```python
from build123d import *

# Parameters (mm, degrees)
SKETCH1_W                 = 50.11
SKETCH1_H                 = 43.44
BOSS_EXTRUDE1_DEPTH       = 97.79
SKETCH2_W                 = 23.32
SKETCH2_H                 = 45.06
CUT_EXTRUDE1_DEPTH        = 119.156378584
SHELL1_T                  = -2
SHELL1_THICKNESS_2_FACE_W = 39.44
SHELL1_THICKNESS_2_FACE_H = 22.79
SHELL1_THICKNESS_2_DEPTH  = 18.02
SKETCH4_W                 = 6.5
SKETCH4_H                 = 11
CUT_EXTRUDE2_DEPTH        = 2
SKETCH6_R                 = 2
CUT_EXTRUDE3_DEPTH        = 2
CUT_EXTRUDE5_DEPTH        = 2
SKETCH8_R                 = 8.25
CUT_EXTRUDE6_DEPTH        = 20.02
FILLET1_R                 = 10
FILLET2_R                 = 2


with BuildPart() as part:
    # Sketch1 → Boss-Extrude1 (new body)
    with BuildSketch(Plane(origin=(0, 0, 0), x_dir=(1, 0, 0), z_dir=(0, 1, 0))):
        with Locations((25.055, 21.72)):
            Rectangle(SKETCH1_W, SKETCH1_H)
    extrude(amount=BOSS_EXTRUDE1_DEPTH)

    # Sketch2 → Cut-Extrude1 (cut, through all)
    with BuildSketch(Plane.XY):
        with Locations((11.66, 22.53)):
            Rectangle(SKETCH2_W, SKETCH2_H)
    extrude(amount=-CUT_EXTRUDE1_DEPTH, mode=Mode.SUBTRACT)

    # Shell1
    shell1_openings = [part.faces().sort_by_distance(p)[0] for p in [
        (25.055, 97.79, -21.72),
    ]]
    offset(amount=SHELL1_T, openings=shell1_openings, kind=Kind.INTERSECTION)

    # Shell1 thickness 2 face (on inner face of the shell) → Shell1 thickness 2 (add)
    with BuildSketch(Plane(origin=(36.715, 2, -21.72), x_dir=(0, 0, -1), z_dir=(0, -1, 0))):
        Rectangle(SHELL1_THICKNESS_2_FACE_W, SHELL1_THICKNESS_2_FACE_H)
    extrude(amount=-SHELL1_THICKNESS_2_DEPTH)

    # Sketch4 → Cut-Extrude2 (cut)
    with BuildSketch(Plane.XZ.offset(-45.06)):
        with Locations((4.35, -30.69)):
            Rectangle(SKETCH4_W, SKETCH4_H)
    extrude(amount=-CUT_EXTRUDE2_DEPTH, mode=Mode.SUBTRACT)

    # Sketch6 → Cut-Extrude3 (cut)
    with BuildSketch(Plane.XY):
        with Locations((44.415, 88.885)):
            Circle(SKETCH6_R)
        with Locations((25.815, 88.885)):
            Circle(SKETCH6_R)
        with Locations((44.415, 53.805)):
            Circle(SKETCH6_R)
        with Locations((25.815, 53.805)):
            Circle(SKETCH6_R)
    extrude(amount=-CUT_EXTRUDE3_DEPTH, mode=Mode.SUBTRACT)

    # Sketch7 → Cut-Extrude5 (cut)
    with BuildSketch(Plane(origin=(0, 0, 0), x_dir=(0, 0, -1), z_dir=(1, 0, 0))):
        with BuildLine():
            Line((22.64, 91.29), (22.64, 97.79))
            Line((22.64, 97.79), (11.64, 97.79))
            Line((11.64, 97.79), (11.64, 91.29))
            ThreePointArc((11.64, 91.29), (17.14, 85.79), (22.64, 91.29))
        make_face()
    extrude(amount=CUT_EXTRUDE5_DEPTH, mode=Mode.SUBTRACT)

    # Sketch8 → Cut-Extrude6 (cut)
    with BuildSketch(Plane(origin=(0, 0, 0), x_dir=(1, 0, 0), z_dir=(0, 1, 0))):
        with Locations(Location((36.715, 21.72, 0), (0, 0, 90))):
            Circle(SKETCH8_R)
    extrude(amount=CUT_EXTRUDE6_DEPTH, mode=Mode.SUBTRACT)

    # Fillet1
    fillet1_edges = [part.edges().sort_by_distance(p)[0] for p in [
        (23.32, 45.06, -21.72),
    ]]
    fillet(fillet1_edges, radius=FILLET1_R)

    # Fillet2
    # the kernel refuses this fillet: 2 mm, written as the material it takes off along each edge
    with BuildSketch(Plane(origin=(2, 47.06, -2), x_dir=(0, -1, 0), z_dir=(0, 0, 1))) as fillet2_piece_1_section:
        Polygon((0, 0), (FILLET2_R, 0), (FILLET2_R, -FILLET2_R), (0, -FILLET2_R), align=None)
    fillet2_piece_1 = extrude(amount=FILLET2_R, mode=Mode.PRIVATE)
    fillet2_piece_1 = fillet2_piece_1 - Plane(origin=(2, 47.06, -2), x_dir=(0.7071067811865475, 0.7071067811865475, 0), z_dir=(0, 0, 1)) * Sphere(FILLET2_R, mode=Mode.PRIVATE)
    add(fillet2_piece_1, mode=Mode.SUBTRACT)
    with BuildSketch(Plane(origin=(2, 47.06, -41.44), x_dir=(-1, 0, 0), z_dir=(0, -1, 0))) as fillet2_piece_2_section:
        Polygon((0, 0), (FILLET2_R, 0), (FILLET2_R, FILLET2_R), (0, FILLET2_R), align=None)
    fillet2_piece_2 = extrude(amount=FILLET2_R, mode=Mode.PRIVATE)
    fillet2_piece_2 = fillet2_piece_2 - Plane(origin=(2, 47.06, -41.44), x_dir=(0.7071067811865475, 0, 0.7071067811865475), z_dir=(0, -1, 0)) * Sphere(FILLET2_R, mode=Mode.PRIVATE)
    add(fillet2_piece_2, mode=Mode.SUBTRACT)
    with BuildSketch(Plane(origin=(2, 95.79, -2), x_dir=(-1, 0, 0), z_dir=(0, 0, 1))) as fillet2_piece_3_section:
        Polygon((0, 0), (FILLET2_R, 0), (FILLET2_R, -FILLET2_R), (0, -FILLET2_R), align=None)
    fillet2_piece_3 = extrude(amount=FILLET2_R, mode=Mode.PRIVATE)
    fillet2_piece_3 = fillet2_piece_3 - Plane(origin=(2, 95.79, -2), x_dir=(0.7071067811865475, -0.7071067811865475, 0), z_dir=(0, 0, 1)) * Sphere(FILLET2_R, mode=Mode.PRIVATE)
    add(fillet2_piece_3, mode=Mode.SUBTRACT)
    with BuildSketch(Plane(origin=(2, 95.79, -41.44), x_dir=(0, 0, -1), z_dir=(-1, 0, 0))) as fillet2_piece_4_section:
        Polygon((0, 0), (FILLET2_R, 0), (FILLET2_R, -FILLET2_R), (0, -FILLET2_R), align=None)
    fillet2_piece_4 = extrude(amount=FILLET2_R, mode=Mode.PRIVATE)
    fillet2_piece_4 = fillet2_piece_4 - Plane(origin=(2, 95.79, -41.44), x_dir=(0, -0.7071067811865475, 0.7071067811865475), z_dir=(-1, 0, 0)) * Sphere(FILLET2_R, mode=Mode.PRIVATE)
    add(fillet2_piece_4, mode=Mode.SUBTRACT)
    with BuildSketch(Plane(origin=(25.32, 2, -2), x_dir=(-1, 0, 0), z_dir=(0, 0, 1))) as fillet2_piece_5_section:
        Polygon((0, 0), (FILLET2_R, 0), (FILLET2_R, FILLET2_R), (0, FILLET2_R), align=None)
    fillet2_piece_5 = extrude(amount=FILLET2_R, mode=Mode.PRIVATE)
    fillet2_piece_5 = fillet2_piece_5 - Plane(origin=(25.32, 2, -2), x_dir=(0.7071067811865475, 0.7071067811865475, 0), z_dir=(0, 0, 1)) * Sphere(FILLET2_R, mode=Mode.PRIVATE)
    add(fillet2_piece_5, mode=Mode.SUBTRACT)
    with BuildSketch(Plane(origin=(25.32, 2, -41.44), x_dir=(0, 0, -1), z_dir=(-1, 0, 0))) as fillet2_piece_6_section:
        Polygon((0, 0), (FILLET2_R, 0), (FILLET2_R, FILLET2_R), (0, FILLET2_R), align=None)
    fillet2_piece_6 = extrude(amount=FILLET2_R, mode=Mode.PRIVATE)
    fillet2_piece_6 = fillet2_piece_6 - Plane(origin=(25.32, 2, -41.44), x_dir=(0, 0.7071067811865475, 0.7071067811865475), z_dir=(-1, 0, 0)) * Sphere(FILLET2_R, mode=Mode.PRIVATE)
    add(fillet2_piece_6, mode=Mode.SUBTRACT)
    with BuildSketch(Plane(origin=(48.11, 2, -2), x_dir=(0, -1, 0), z_dir=(0, 0, 1))) as fillet2_piece_7_section:
        Polygon((0, 0), (FILLET2_R, 0), (FILLET2_R, FILLET2_R), (0, FILLET2_R), align=None)
    fillet2_piece_7 = extrude(amount=FILLET2_R, mode=Mode.PRIVATE)
    fillet2_piece_7 = fillet2_piece_7 - Plane(origin=(48.11, 2, -2), x_dir=(-0.7071067811865475, 0.7071067811865475, 0), z_dir=(0, 0, 1)) * Sphere(FILLET2_R, mode=Mode.PRIVATE)
    add(fillet2_piece_7, mode=Mode.SUBTRACT)
    with BuildSketch(Plane(origin=(48.11, 95.79, -2), x_dir=(0, 1, 0), z_dir=(0, 0, 1))) as fillet2_piece_8_section:
        Polygon((0, 0), (FILLET2_R, 0), (FILLET2_R, -FILLET2_R), (0, -FILLET2_R), align=None)
    fillet2_piece_8 = extrude(amount=FILLET2_R, mode=Mode.PRIVATE)
    fillet2_piece_8 = fillet2_piece_8 - Plane(origin=(48.11, 95.79, -2), x_dir=(-0.7071067811865475, -0.7071067811865475, 0), z_dir=(0, 0, 1)) * Sphere(FILLET2_R, mode=Mode.PRIVATE)
    add(fillet2_piece_8, mode=Mode.SUBTRACT)
    with BuildSketch(Plane(origin=(48.11, 95.79, -41.44), x_dir=(0, 1, 0), z_dir=(0, 0, -1))) as fillet2_piece_9_section:
        Polygon((0, 0), (FILLET2_R, 0), (FILLET2_R, FILLET2_R), (0, FILLET2_R), align=None)
    fillet2_piece_9 = extrude(amount=FILLET2_R, mode=Mode.PRIVATE)
    fillet2_piece_9 = fillet2_piece_9 - Plane(origin=(48.11, 95.79, -41.44), x_dir=(-0.7071067811865475, -0.7071067811865475, 0), z_dir=(0, 0, -1)) * Sphere(FILLET2_R, mode=Mode.PRIVATE)
    add(fillet2_piece_9, mode=Mode.SUBTRACT)
    with BuildSketch(Plane(origin=(48.11, 2, -41.44), x_dir=(0, -1, 0), z_dir=(0, 0, -1))) as fillet2_piece_10_section:
        Polygon((0, 0), (FILLET2_R, 0), (FILLET2_R, -FILLET2_R), (0, -FILLET2_R), align=None)
    fillet2_piece_10 = extrude(amount=FILLET2_R, mode=Mode.PRIVATE)
    fillet2_piece_10 = fillet2_piece_10 - Plane(origin=(48.11, 2, -41.44), x_dir=(-0.7071067811865475, 0.7071067811865475, 0), z_dir=(0, 0, -1)) * Sphere(FILLET2_R, mode=Mode.PRIVATE)
    add(fillet2_piece_10, mode=Mode.SUBTRACT)
    with BuildSketch(Plane(origin=(0, 45.06, -2), x_dir=(1, 0, 0), z_dir=(0, 0, -1)), Plane(origin=(50.11, 97.79, -2), x_dir=(-1, 0, 0), z_dir=(0, 0, -1))) as fillet2_piece_11:
        with BuildLine():
            CenterArc((FILLET2_R, -FILLET2_R), FILLET2_R, 90, 90)
            Line((0, -FILLET2_R), (0, 0))
            Line((0, 0), (FILLET2_R, 0))
        make_face()
    extrude(amount=39.44, mode=Mode.SUBTRACT)
    with BuildSketch(Plane(origin=(0, 97.79, -16.64), x_dir=(0, -1, 0), z_dir=(0, 0, 1))) as fillet2_piece_12:
        with BuildLine():
            CenterArc((FILLET2_R, FILLET2_R), FILLET2_R, 180, 90)
            Line((0, FILLET2_R), (0, 0))
            Line((0, 0), (FILLET2_R, 0))
        make_face()
    extrude(amount=14.64, mode=Mode.SUBTRACT)
    with BuildSketch(Plane(origin=(0, 47.06, 0), x_dir=(1, 0, 0), z_dir=(0, 1, 0)), Plane(origin=(0, 47.06, -43.44), x_dir=(0, 0, 1), z_dir=(0, 1, 0))) as fillet2_piece_13:
        with BuildLine():
            CenterArc((FILLET2_R, FILLET2_R), FILLET2_R, 180, 90)
            Line((0, FILLET2_R), (0, 0))
            Line((0, 0), (FILLET2_R, 0))
        make_face()
    extrude(amount=48.73, mode=Mode.SUBTRACT)
    with BuildSketch(Plane(origin=(0, 97.79, -41.44), x_dir=(0, -1, 0), z_dir=(0, 0, 1))) as fillet2_piece_14:
        with BuildLine():
            CenterArc((FILLET2_R, FILLET2_R), FILLET2_R, 180, 90)
            Line((0, FILLET2_R), (0, 0))
            Line((0, 0), (FILLET2_R, 0))
        make_face()
    extrude(amount=23.8, mode=Mode.SUBTRACT)
    with BuildSketch(Plane(origin=(13.32, 45.06, 0), x_dir=(0, 1, 0), z_dir=(-1, 0, 0)), Plane(origin=(13.32, 45.06, -43.44), x_dir=(0, 0, 1), z_dir=(-1, 0, 0))) as fillet2_piece_15:
        with BuildLine():
            CenterArc((FILLET2_R, FILLET2_R), FILLET2_R, 180, 90)
            Line((0, FILLET2_R), (0, 0))
            Line((0, 0), (FILLET2_R, 0))
        make_face()
    extrude(amount=11.32, mode=Mode.SUBTRACT)
    with BuildSketch(Plane(origin=(23.32, 2, 0), x_dir=(1, 0, 0), z_dir=(0, 1, 0)), Plane(origin=(23.32, 2, -43.44), x_dir=(0, 0, 1), z_dir=(0, 1, 0))) as fillet2_piece_16:
        with BuildLine():
            CenterArc((FILLET2_R, FILLET2_R), FILLET2_R, 180, 90)
            Line((0, FILLET2_R), (0, 0))
            Line((0, 0), (FILLET2_R, 0))
        make_face()
    extrude(amount=33.06, mode=Mode.SUBTRACT)
    with BuildSketch(Plane(origin=(50.11, 2, 0), x_dir=(-1, 0, 0), z_dir=(0, 1, 0)), Plane(origin=(50.11, 2, -43.44), x_dir=(0, 0, 1), z_dir=(0, 1, 0))) as fillet2_piece_17:
        with BuildLine():
            CenterArc((FILLET2_R, -FILLET2_R), FILLET2_R, 90, 90)
            Line((0, -FILLET2_R), (0, 0))
            Line((0, 0), (FILLET2_R, 0))
        make_face()
    extrude(amount=93.79, mode=Mode.SUBTRACT)
    with BuildSketch(Plane(origin=(25.32, 0, 0), x_dir=(0, 1, 0), z_dir=(1, 0, 0))) as fillet2_piece_18:
        with BuildLine():
            CenterArc((FILLET2_R, -FILLET2_R), FILLET2_R, 90, 90)
            Line((0, -FILLET2_R), (0, 0))
            Line((0, 0), (FILLET2_R, 0))
        make_face()
    extrude(amount=22.79, mode=Mode.SUBTRACT)
    with BuildSketch(Plane(origin=(50.11, 0, -2), x_dir=(-1, 0, 0), z_dir=(0, 0, -1)), Plane(origin=(23.32, 0, -2), x_dir=(0, 1, 0), z_dir=(0, 0, -1))) as fillet2_piece_19:
        with BuildLine():
            CenterArc((FILLET2_R, FILLET2_R), FILLET2_R, 180, 90)
            Line((0, FILLET2_R), (0, 0))
            Line((0, 0), (FILLET2_R, 0))
        make_face()
    extrude(amount=39.44, mode=Mode.SUBTRACT)
    with BuildSketch(Plane(origin=(48.11, 0, -43.44), x_dir=(0, 0, 1), z_dir=(-1, 0, 0))) as fillet2_piece_20:
        with BuildLine():
            CenterArc((FILLET2_R, FILLET2_R), FILLET2_R, 180, 90)
            Line((0, FILLET2_R), (0, 0))
            Line((0, 0), (FILLET2_R, 0))
        make_face()
    extrude(amount=22.79, mode=Mode.SUBTRACT)
    with BuildSketch(Plane(origin=(13.32, 35.06, 0), x_dir=(0, 1, 0), z_dir=(-1, 0, 0))) as fillet2_piece_21:
        with BuildLine():
            CenterArc((10 + FILLET2_R, FILLET2_R), FILLET2_R, 180, 90)
            Line((10, FILLET2_R), (10, 0))
            Line((10, 0), (10 + FILLET2_R, 0))
        make_face()
    revolve(axis=Axis((13.32, 35.06, 0), (0, 0, -1)), revolution_arc=90, mode=Mode.SUBTRACT)
    with BuildSketch(Plane(origin=(13.32, 35.06, -43.44), x_dir=(0, 1, 0), z_dir=(-1, 0, 0))) as fillet2_piece_22:
        with BuildLine():
            CenterArc((10 + FILLET2_R, -FILLET2_R), FILLET2_R, 90, 90)
            Line((10 + FILLET2_R, 0), (10, 0))
            Line((10, 0), (10, -FILLET2_R))
        make_face()
    revolve(axis=Axis((13.32, 35.06, -43.44), (0, 0, -1)), revolution_arc=90, mode=Mode.SUBTRACT)
    with BuildSketch(Plane(origin=(2, 97.79, 0), x_dir=(0, -1, 0), z_dir=(1, 0, 0))) as fillet2_piece_23:
        with BuildLine():
            CenterArc((FILLET2_R, FILLET2_R), FILLET2_R, 180, 90)
            Line((0, FILLET2_R), (0, 0))
            Line((0, 0), (FILLET2_R, 0))
        make_face()
    extrude(amount=46.11, mode=Mode.SUBTRACT)
    with BuildSketch(Plane(origin=(48.11, 97.79, -43.44), x_dir=(0, 0, 1), z_dir=(-1, 0, 0))) as fillet2_piece_24:
        with BuildLine():
            CenterArc((FILLET2_R, -FILLET2_R), FILLET2_R, 90, 90)
            Line((0, -FILLET2_R), (0, 0))
            Line((0, 0), (FILLET2_R, 0))
        make_face()
    extrude(amount=46.11, mode=Mode.SUBTRACT)


solid = part.part
```
Geometry check sheet. Reference: the model listing, model coordinates, mm. A direction names the side the tool comes from. Round coordinates to 2 decimals unless told otherwise and drop trailing zeros. Order: outer loops, then holes, each group sorted by start corner. A loop starts at its lowest first (then second) coordinate and runs counter-clockwise, first axis right, second up. Notation, with made-up numbers: (27, 58) - (64, 58) arc R18 cw to (64, 72) - close; hole circle Ø4 at (66, 60.5). An arc over 180 degrees is marked (long way). Use a Markdown table: item, result. Add a question column.
1) Set-up check for faces 1 (the cylindrical face through (7.74, 45.63, -0.6)), 2 (the flat face through (1.1, 46, -31)), 3 (the flat face through (1, 94, -22.64)): record each of +Z, -Z, +X, -X, +Y, -Y from which the full face is reachable in a straight line by a thin tool's end or side.
2) Mould release check, pull along Z, two halves, no side actions. Record for faces 4 (the cylindrical face through (41.73, 9.87, -15.17)), 5 (the flat face through (36.9, 20.02, -30.2)), 6 (the cylindrical face through (42.828, 52.588, -0.986)), 7 (the cylindrical face through (0.57, 71.08, -0.6)): released by +Z, released by -Z, zero draft, split by the parting line, or undercut.
3) Gauge pin test, flat ends, axial feed: P1, Ø1, axis at x = 36, z = -38, coming from the +Y side; P2, Ø3, axis at x = 11.5, z = -12, coming from the +Y side; P3, Ø0.6, axis at y = 46, z = -31, coming from the -X side. Record the tip position at first contact, or that the pin passes through.
4) Section check D-D (x = 11). Record the cut outline in (y, z), then the cut area to 3 significant figures.
5) Thickness scan on line 1 along X through (y, z) = (62, -12); line 2 along Z through (x, y) = (22.5, 54.5); line 3 along X through (y, z) = (32, -8). Record the ranges inside material, lowest first.
6) Section check A-A (y = 73). Record the cut outline in (x, z), then the cut area to 3 significant figures.
7) Section check C-C (z = -17.14). Record the cut outline in (x, y).
8) Section check B-B (z = -27). Record the cut outline in (x, y), then the cut area to 3 significant figures.
Established:
| question | item | result |
|---|---|---|
| 1 | face 1 | +Z, -X, -Y |
| 1 | face 2 | -Y |
| 1 | face 3 | -X, +Y |
| 2 | face 4 | undercut |
| 2 | face 5 | undercut |
| 2 | face 6 | zero draft |
| 2 | face 7 | released by +Z |
| 3 | P1 | y = 20.02 |
| 3 | P2 | y = 47.06 |
| 3 | P3 | x = 0.15 |
| 4 | outline | (45.06, -41.44) arc R2 ccw to (47.06, -43.44) - (95.79, -43.44) arc R2 ccw to (97.79, -41.44) - (47.06, -41.44) - (47.06, -2) - (97.79, -2) arc R2 ccw to (95.79, 0) - (47.06, 0) arc R2 ccw to (45.06, -2) - close |
| 4 | area | 286 mm2 |
| 5 | line 1 | 0 to 2, 48.11 to 50.11 |
| 5 | line 2 | -43.44 to -41.44, -2 to 0 |
| 5 | line 3 | 23.32 to 25.32, 48.11 to 50.11 |
| 6 | outline | (0, -41.44) arc R2 ccw to (2, -43.44) - (48.11, -43.44) arc R2 ccw to (50.11, -41.44) - (50.11, -2) arc R2 ccw to (48.11, 0) - (2, 0) arc R2 ccw to (0, -2) - close; hole (2, -41.44) - (48.11, -41.44) - (48.11, -2) - (2, -2) - close |
| 6 | area | 355 mm2 |
| 7 | outline | (0, 47.06) arc R2 ccw to (2, 45.06) - (13.32, 45.06) arc R10 cw to (23.32, 35.06) - (23.32, 2) arc R2 ccw to (25.32, 0) - (29.85, 0) - (29.85, 20.02) - (25.32, 20.02) - (25.32, 47.06) - (2, 47.06) - (2, 85.79) - (0, 85.79) - close; (43.58, 0) - (48.11, 0) arc R2 ccw to (50.11, 2) - (50.11, 95.79) arc R2 ccw to (48.11, 97.79) - (48.11, 20.02) - (43.58, 20.02) - close |
| 8 | outline | (0, 47.06) arc R2 ccw to (1.1, 45.27) - (1.1, 47.06) - (2, 47.06) - (2, 97.79) arc R2 ccw to (0, 95.79) - close; (7.6, 45.06) - (13.32, 45.06) arc R10 cw to (23.32, 35.06) - (23.32, 2) arc R2 ccw to (25.32, 0) - (30.38, 0) - (30.38, 20.02) - (25.32, 20.02) - (25.32, 47.06) - (7.6, 47.06) - close; (43.05, 0) - (48.11, 0) arc R2 ccw to (50.11, 2) - (50.11, 95.79) arc R2 ccw to (48.11, 97.79) - (48.11, 20.02) - (43.05, 20.02) - close |
| 8 | area | 644 mm2 |
